```python
from build123d import *

# Parameters (mm, degrees)
SKETCH1_W           = 125
SKETCH1_H           = 55
BOSS_EXTRUDE1_DEPTH = 3
SKETCH2_W           = 4
SKETCH2_H           = 10
SKETCH2_H_2         = 15
SKETCH2_W_2         = 15
SKETCH2_H_3         = 4
BOSS_EXTRUDE2_DEPTH = 3


with BuildPart() as part:
    # Sketch1 → Boss-Extrude1 (new body)
    with BuildSketch(Plane.XY):
        with Locations((-62.5, 27.5)):
            Rectangle(SKETCH1_W, SKETCH1_H)
    extrude(amount=BOSS_EXTRUDE1_DEPTH)

    # Sketch2 → Boss-Extrude2 (add)
    with BuildSketch(Plane.XY.offset(3)):
        with Locations((-127, 5)):
            Rectangle(SKETCH2_W, SKETCH2_H)
        with Locations((2, 5)):
            Rectangle(SKETCH2_W, SKETCH2_H)
        with Locations((2, 32.5)):
            Rectangle(SKETCH2_W, SKETCH2_H_2)
        with Locations((-127, 32.5)):
            Rectangle(SKETCH2_W, SKETCH2_H_2)
        with Locations((-72.5, 57)):
            Rectangle(SKETCH2_W_2, SKETCH2_H_3)
        with Locations((-22.5, 57)):
            Rectangle(SKETCH2_W_2, SKETCH2_H_3)
        with Locations((-102.5, 57)):
            Rectangle(SKETCH2_W_2, SKETCH2_H_3)
        with Locations((-52.5, 57)):
            Rectangle(SKETCH2_W_2, SKETCH2_H_3)
    extrude(amount=-BOSS_EXTRUDE2_DEPTH)


solid = part.part
```
Can you work these out from the model? Positions are in its coordinate system, mm. A direction names the side the tool comes from. Coordinates: 2 decimals unless noted, no trailing zeros. Loops run counter-clockwise (first coordinate to the right, second up) from the corner with the lowest first, then second, coordinate; pieces in that order, holes last.
1) Imagine slicing it at B-B on x = -39. List the corners of the cut face in (y, z) for me.
2) Imagine slicing it at C-C on y = 47.5. List the corners of the cut face in (x, z) for me, plus the area to 3 significant figures.
3) For pin 1 (0.9 mm diameter, centred on x = -119, z = 1.5, fed in from +Y); pin 2 (0.9 mm diameter, centred on y = 57, z = 1.5, fed in from -X); pin 3 (0.9 mm diameter, centred on y = 56.5, z = 1.5, fed in from +X), each with a flat end and sliding along its axis, tell me the tip position at first contact or that it passes through.
4) Which directions (+Z, -Z, +X, -X, +Y, -Y) give clear straight access to the entire face, cutting with the end or side of a thin tool? Please do faces 4 (the flat face through (-30, 57, 2)), 5 (the flat face through (0, 17, 1)), 6 (the flat face through (-125, 47, 1)), 7 (the flat face through (-8, 55, 1)).
5) I need wall thicknesses on probe 1 along Y at (x, z) = (-13.5, 0.4); probe 2 along X at (y, z) = (17, 1). Which ranges of each line are inside material? Lowest first, please.
6) Thinking about a two-plate mould opening in Y: for faces 1 (the flat face through (2, 10, 2)), 2 (the flat face through (-73, 59, 2)), 3 (the flat face through (-129, 32, 2)), which applies, pulls with the +Y half, pulls with the -Y half, needs draft (parallel to the pull), parting line crosses it, or undercut?
Completed:
1. outline: (0, 0) - (55, 0) - (55, 3) - (0, 3) - close
2. outline: (-125, 0) - (0, 0) - (0, 3) - (-125, 3) - close
2. area: 375 mm2
3. pin 1: stops at y = 55
3. pin 2: stops at x = -110
3. pin 3: stops at x = -15
4. face 4: +Z, -Z, +Y
4. face 5: +Z, -Z, +X
4. face 6: +Z, -Z, -X, +Y
4. face 7: +Z, -Z, +X, +Y
5. probe 1: y = 0 to 55
5. probe 2: x = -125 to 0
6. face 1: undercut
6. face 2: pulls with the +Y half
6. face 3: needs draft
